from build123d import *

# Parameters (mm, degrees)
SKETCH1_W               = 99
SKETCH1_H               = 69.5
BOSS_EXTRUDE1_DEPTH     = 1.6
SKETCH2_R               = 5.1
BOSS_EXTRUDE2_DEPTH     = 17
SKETCH3_R               = 1.4
SKETCH3_R_2             = 1.65
SKETCH3_R_3             = 0.45
CUT_EXTRUDE1_DEPTH      = 18
CUT_EXTRUDE1_DEPTH_BACK = 2.6


with BuildPart() as part:
    # Sketch1 → Boss-Extrude1 (new body)
    with BuildSketch(Plane.XY):
        with Locations((49.5, 34.75)):
            Rectangle(SKETCH1_W, SKETCH1_H)
    extrude(amount=BOSS_EXTRUDE1_DEPTH)

    # Sketch2 → Boss-Extrude2 (add)
    with BuildSketch(Plane.XY.offset(1.6)):
        with Locations((18, 48)):
            Circle(SKETCH2_R)
        with Locations((30, 48)):
            Circle(SKETCH2_R)
        with Locations((69, 48)):
            Circle(SKETCH2_R)
        with Locations((81, 48)):
            Circle(SKETCH2_R)
    extrude(amount=BOSS_EXTRUDE2_DEPTH)

    # Sketch3 → Cut-Extrude1 (cut, two sides)
    with BuildSketch(Plane.XY.offset(1.6)) as cut_extrude1_sk:
        with Locations((10, 67.1)):
            Circle(SKETCH3_R)
        with Locations((89, 67.1)):
            Circle(SKETCH3_R)
        with Locations((18.5, 15)):
            Circle(SKETCH3_R_2)
        with Locations((77, 15)):
            Circle(SKETCH3_R_2)
        with Locations((49.5, 48.5)):
            Circle(SKETCH3_R_3)
        with Locations((52.06, 48.5)):
            Circle(SKETCH3_R_3)
        with Locations((46.94, 48.5)):
            Circle(SKETCH3_R_3)
        with Locations((43.15, 3)):
            Circle(SKETCH3_R_3)
        with Locations((45.69, 3)):
            Circle(SKETCH3_R_3)
        with Locations((48.23, 3)):
            Circle(SKETCH3_R_3)
        with Locations((50.77, 3)):
            Circle(SKETCH3_R_3)
        with Locations((53.31, 3)):
            Circle(SKETCH3_R_3)
        with Locations((55.85, 3)):
            Circle(SKETCH3_R_3)
        with Locations((58.39, 3)):
            Circle(SKETCH3_R_3)
        with Locations((60.93, 3)):
            Circle(SKETCH3_R_3)
        with Locations((40.61, 3)):
            Circle(SKETCH3_R_3)
        with Locations((38.07, 3)):
            Circle(SKETCH3_R_3)
    extrude(amount=CUT_EXTRUDE1_DEPTH, mode=Mode.SUBTRACT)
    extrude(cut_extrude1_sk.sketch, amount=-CUT_EXTRUDE1_DEPTH_BACK, mode=Mode.SUBTRACT)


solid = part.part
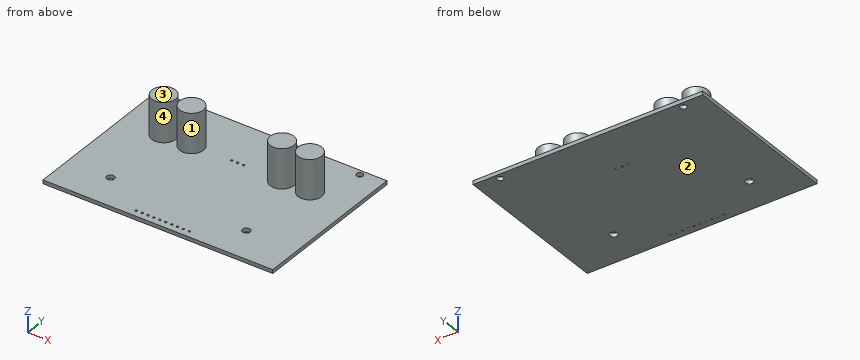
For this review, take the finished solid that the model builds, in its own axes (mm). Face numbers are marked on the shaded views. A direction names the side the tool comes from. Give positions to 0.01 mm unless a question says otherwise; leave off trailing zeros. Loops run counter-clockwise (first coordinate to the right, second up) from the corner with the lowest first, then second, coordinate; pieces in that order, holes last. Notation, with made-up numbers: (69, 18) -> (126, 18) arc R19 cw to (126, 22) -> close; hole circle Ø9 at (16.5, 42.25). An arc over 180 degrees is marked (long way). One line per question, with ' | ' between items.
1) We need section C-C (x = 69). Write out the cut boundary in (y, z), plus the area to 3 significant figures.
Resolved:
outline: (0, 0) -> (69.5, 0) -> (69.5, 1.6) -> (53.1, 1.6) -> (53.1, 18.6) -> (42.9, 18.6) -> (42.9, 1.6) -> (0, 1.6) -> close | area: 285 mm2
2) We need section D-D (y = 33.5). Write out the cut boundary in (x, z).
Resolved:
outline: (0, 0) -> (99, 0) -> (99, 1.6) -> (0, 1.6) -> close
3) We need section A-A (x = 18). Write out the cut boundary in (y, z), plus the area to 3 significant figures.
Resolved:
outline: (0, 0) -> (13.43, 0) -> (13.43, 1.6) -> (0, 1.6) -> close; (16.57, 0) -> (69.5, 0) -> (69.5, 1.6) -> (53.1, 1.6) -> (53.1, 18.6) -> (42.9, 18.6) -> (42.9, 1.6) -> (16.57, 1.6) -> close | area: 280 mm2
4) The part is to be moulded in two halves that separate along X. For the marked faces 3 and 4, say which applies: +X half, -X half, draft (parallel to the pull), parting line (faces both ways), or undercut.
Resolved:
face 3: draft | face 4: undercut
5) We need section B-B (z = 10.25). Write out the cut boundary in (x, y).
Resolved:
outline: circle Ø10.2 at (18, 48); circle Ø10.2 at (30, 48); circle Ø10.2 at (69, 48); circle Ø10.2 at (81, 48)
6) For the marked faces 1 and 2, list the 3-axis set-ups (+Z, -Z, +X, -X, +Y, -Y) from which the entire face can be reached by the end or side of a thin tool; tool diameter is ignored.
Resolved:
face 1: +Z | face 2: -Z, +X, -X, +Y, -Y
7) Insertion check: pin 1 Ø12 at (x, y) = (35.5, 23) entering from +Z; pin 2 Ø4 at (x, z) = (80, 14.5) entering from +Y. Each pin has a flat end and moves straight along its axis. Give the tip position at first contact, or say it passes through.
Resolved:
pin 1: stops at z = 1.6 | pin 2: stops at y = 53.1
8) To check wall thickness, follow probe 1 along X at (y, z) = (48.5, 0.65); probe 2 along X at (y, z) = (67.1, 1.1); probe 3 along Y at (x, z) = (58.39, 0.45). State the ranges of each line that lie inside material, in increasing order.
Resolved:
probe 1: x = 0 to 46.49, 47.39 to 49.05, 49.95 to 51.61, 52.51 to 99 | probe 2: x = 0 to 8.6, 11.4 to 87.6, 90.4 to 99 | probe 3: y = 0 to 2.55, 3.45 to 69.5
